For this review, take the finished solid that the model builds, in its own axes (mm). A direction names the side the tool comes from. Coordinates: 2 decimals unless noted, no trailing zeros. Loops run counter-clockwise (first coordinate to the right, second up) from the corner with the lowest first, then second, coordinate; pieces in that order, holes last. Notation, with made-up numbers: (53.25, -18.5) - (103.25, -18.5) arc R24 ccw to (103.25, 10.5) - close; hole circle Ø11 at (29.5, -36). An arc over 180 degrees is marked (long way). Answer as a JSON object with one key per item and string values. Group by question number.
Item 1: Tool access review of faces 5 (the flat face through (28, 58.2, -5)), 6 (the flat face through (48, 50, 8)), 7 (the flat face through (49, 49, -5)), 8 (the flat face through (7.5, 49, -5)): name each direction out of +Z, -Z, +X, -X, +Y, -Y from which nothing blocks a thin tool from reaching the whole face with its end or side.
Item 2: We need section D-D (z = -7.75). Give the boundary of the cut face in (x, y).
Item 3: Mouldability with a two-part tool opening along X and no side actions: class faces 1 (the cylindrical face through (2.34, 56.46, 1.38)), 2 (the flat face through (50, 60.2, 1)), 3 (the flat face through (97.8, 30, 8)), 4 (the cylindrical face through (96.99, 2.12, 1.38)) as released by +X, released by -X, zero draft, split by the parting line, or undercut.
Item 4: To check wall thickness, follow line 1 (Y direction, x = 95.8, z = 0.6); line 2 (Y direction, x = 67.5, z = 11.5); line 3 (X direction, y = 11, z = 11.5). State the ranges of each line that lie inside material, in increasing order.
Item 5: We need section B-B (y = 2.5). Give the boundary of the cut face in (x, z).
Item 6: We need section C-C (x = 75). Give the boundary of the cut face in (y, z).
Item 7: Clearance check with flat-ended pins moving along their axes: pin 1 (10 mm diameter, centred on x = 20.5, y = 26.5, fed in from +Z); pin 2 (5 mm diameter, centred on x = 27, z = -7.5, fed in from -Y); pin 3 (10 mm diameter, centred on x = 29.5, y = 12.5, fed in from -Z); pin 4 (11 mm diameter, centred on x = 34.5, z = 6.5, fed in from -Y). State where each tip first meets the part, or that it passes through.
Item 8: We need section A-A (x = 95.8). Give the boundary of the cut face in (y, z), then the cut area to 3 significant figures.
Autodesk Inventor part; units mm, degrees
ref_plane "YZ Plane" through (0, 0, 0) normal (1, 0, 0) x (0, 1, 0)
ref_plane "XZ Plane" through (0, 0, 0) normal (0, 1, 0) x (-1, 0, 0)
ref_plane "XY Plane" through (0, 0, 0) normal (0, 0, 1) x (1, 0, 0)
sketch "Sketch1" plane through (0, 0, 0) normal (0, 0, 1) x (1, 0, 0)
  line L0 (0, 0) -> (98.3, 0)
  line L1 (98.3, 0) -> (98.3, 60.2)
  line L2 (98.3, 60.2) -> (0, 60.2)
  line L3 (0, 60.2) -> (0, 0)
  line L4 (0, 60.2) -> (2.5, 60.2) construction
  line L5 (2.5, 60.2) -> (2.5, 57.7) construction
  line L6 (2.5, 57.7) -> (0, 57.7) construction
  line L7 (0, 57.7) -> (0, 60.2) construction
  circle A0 centre (2.5, 57.7) radius 1.25
  line L8 (49.15, 60.2) -> (49.15, 0) construction
  line L9 (0, 30.1) -> (98.3, 30.1) construction
  circle A1 centre (95.8, 57.7) radius 1.25
  circle A2 centre (2.5, 2.5) radius 1.25
  circle A3 centre (95.8, 2.5) radius 1.25
  dimension "d0" = 98.3
  dimension "d1" = 60.2
  dimension "d2" = 2.5
  dimension "d7" = 2.5
  dimension "d8" = 2.5
extrude "LcdPcb" add sketch "Sketch1" along normal blind 2.8
sketch "Sketch2" plane through (0, 0, 2.8) normal (0, 0, 1) x (1, 0, 0)
  line L0 (98.3, 60.2) -> (0, 60.2) construction
  line L1 (49.15, 60.2) -> (49.15, 0) construction
  line L2 (0, 0) -> (98.3, 0) construction
  line L3 (0, 60.2) -> (0, 0) construction
  line L4 (0, 30.1) -> (98.3, 30.1) construction
  line L5 (98.3, 0) -> (98.3, 60.2) construction
  line L6 (0.5, 50) -> (97.8, 50)
  line L7 (97.8, 50) -> (97.8, 10.2)
  line L8 (97.8, 10.2) -> (0.5, 10.2)
  line L9 (0.5, 10.2) -> (0.5, 50)
  line L10 (0.5, 50) -> (97.8, 10.2) construction
  line L11 (97.8, 50) -> (0.5, 10.2) construction
  point P0 (49.15, 30.1)
  dimension "d15" = 39.8
  dimension "d16" = 97.3
extrude "LcdBezel" add sketch "Sketch2" along normal blind 9.9
sketch "Sketch3" plane through (0, 0, 12.7) normal (0, 0, 1) x (1, 0, 0)
  line L0 (0.5, 50) -> (0.5, 10.2) construction
  line L1 (0.5, 50) -> (11.3, 50) construction
  line L2 (11.3, 50) -> (11.3, 43.1) construction
  line L3 (11.3, 43.1) -> (0.5, 43.1) construction
  line L4 (0.5, 43.1) -> (0.5, 50) construction
  line L5 (11.3, 43.1) -> (87, 43.1)
  line L6 (87, 43.1) -> (87, 17.1)
  line L7 (87, 17.1) -> (11.3, 17.1)
  line L8 (11.3, 17.1) -> (11.3, 43.1)
  point P0 (0, 0)
  dimension "LcdBezelHeight" = 6.9
  dimension "LcdBezelLength" = 10.8
  dimension "d28" = 75.7
  dimension "d29" = 26
extrude "Lcd" cut sketch "Sketch3" against normal blind 1.4
sketch "Sketch4" plane through (0, 0, 0) normal (0, 0, -1) x (-1, 0, 0)
  line L0 (0, 60.2) -> (0, 0) construction
  line L1 (0, 60.2) -> (-7.5, 60.2) construction
  line L2 (-7.5, 60.2) -> (-7.5, 58.2) construction
  line L3 (-7.5, 58.2) -> (0, 58.2) construction
  line L4 (0, 58.2) -> (0, 60.2) construction
  line L5 (-7.5, 58.2) -> (-49, 58.2)
  line L6 (-49, 58.2) -> (-49, 39.2)
  line L7 (-49, 39.2) -> (-7.5, 39.2)
  line L8 (-7.5, 39.2) -> (-7.5, 58.2)
  dimension "LcdRearKeepOutHeightOffset" = 2
  dimension "LcdRearKeepOutLengthOffset" = 7.5
  dimension "LcdRearKeepOutHeight" = 19
  dimension "LcdRearKeepOutLength" = 41.5
extrude "LcdRearKeepOut" add sketch "Sketch4" along normal blind 10
equation "\"d0\" = LcdBorderLength"
equation "\"d1\" = LcdBorderHeight"
equation "\"d2\" = LcdFrameHoleOffset"
equation "\"d7\" = LcdFrameHoleOffset"
equation "\"d8\" = LcdFrameHoleDiameterUntapped"
equation "\"d12\" = LcdPcbThickness"
equation "\"d15\" = LcdHeight"
equation "\"d16\" = LcdLength"
equation "\"d28\" = LcdLength - 2 * LcdBezelLength"
equation "\"d29\" = LcdHeight - 2 * LcdBezelHeight"
equation "\"d30\" = 0.5 * LcdPcbThickness"
properties part number "2020-04-12 LcdAssembly"
Check sheet entries:
{
 "1": {"face 5": "-Z, +X, -X, +Y", "face 6": "+Z, +X, -X, +Y", "face 7": "-Z, +X, +Y, -Y", "face 8": "-Z, -X, +Y, -Y"},
 "2": {"outline": "(7.5, 39.2) - (49, 39.2) - (49, 58.2) - (7.5, 58.2) - close"},
 "3": {"face 1": "undercut", "face 2": "zero draft", "face 3": "released by +X", "face 4": "undercut"},
 "4": {"line 1": "y = 0 to 1.25, 3.75 to 56.45, 58.95 to 60.2", "line 2": "y = 10.2 to 17.1, 43.1 to 50", "line 3": "x = 0.5 to 97.8"},
 "5": {"outline": "(0, 0) - (1.25, 0) - (1.25, 2.8) - (0, 2.8) - close; (3.75, 0) - (94.55, 0) - (94.55, 2.8) - (3.75, 2.8) - close; (97.05, 0) - (98.3, 0) - (98.3, 2.8) - (97.05, 2.8) - close"},
 "6": {"outline": "(0, 0) - (60.2, 0) - (60.2, 2.8) - (50, 2.8) - (50, 12.7) - (43.1, 12.7) - (43.1, 11.3) - (17.1, 11.3) - (17.1, 12.7) - (10.2, 12.7) - (10.2, 2.8) - (0, 2.8) - close"},
 "7": {"pin 1": "stops at z = 11.3", "pin 2": "stops at y = 39.2", "pin 3": "stops at z = 0", "pin 4": "stops at y = 0"},
 "8": {"outline": "(0, 0) - (1.25, 0) - (1.25, 2.8) - (0, 2.8) - close; (3.75, 0) - (56.45, 0) - (56.45, 2.8) - (50, 2.8) - (50, 12.7) - (10.2, 12.7) - (10.2, 2.8) - (3.75, 2.8) - close; (58.95, 0) - (60.2, 0) - (60.2, 2.8) - (58.95, 2.8) - close", "area": "549 mm2"}
}
